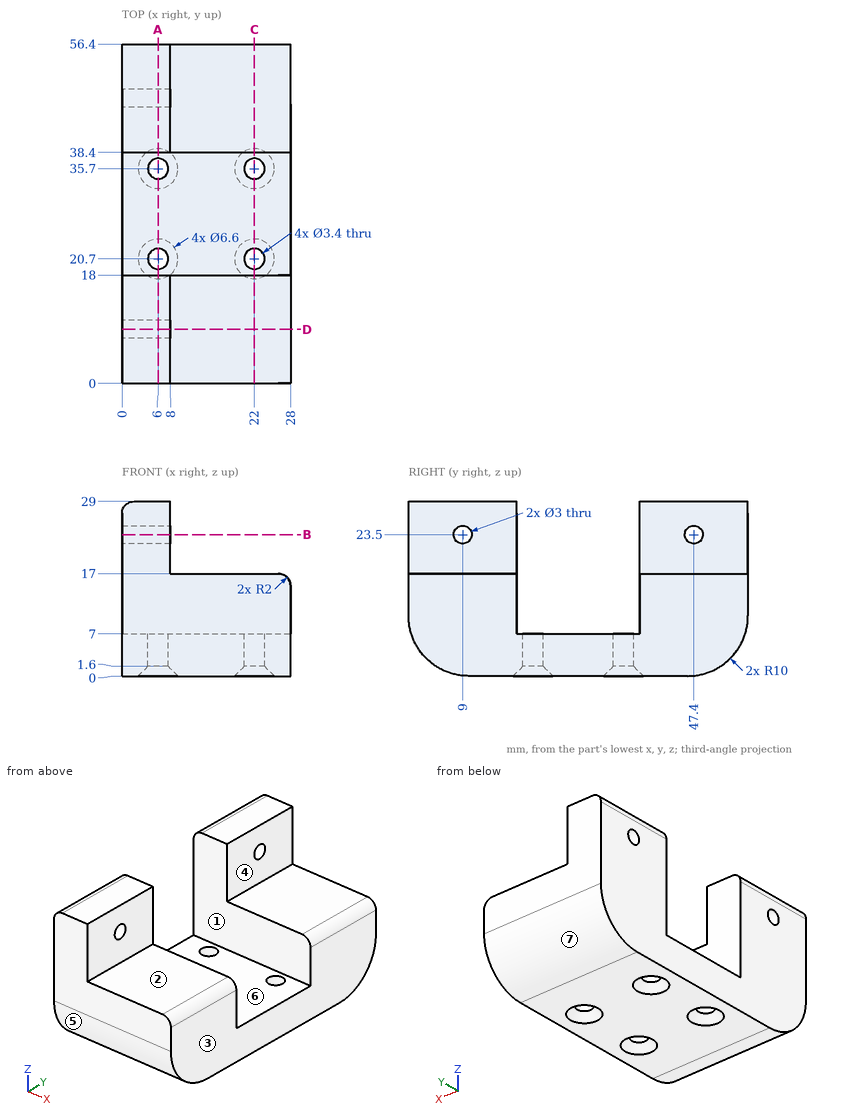
Drawing for the job (mm, zero at the part's lowest x, y, z). A direction names the side the tool comes from. Round coordinates to 2 decimals unless told otherwise and drop trailing zeros. Write each loop counter-clockwise with the first axis right and the second up, starting at its lowest first coordinate (ties: lowest second). Pieces come first, ordered by that corner, then holes. Notation, with made-up numbers: M 74.5,49 L 128.5,49 A7 ccw 128.5,54 Z; hole C 26,69.25 d2. An arc over 180 degrees is marked long. Put each result on its own line as item: value.
Item 1: Cut at D-D (y = 9). List the corners of the cut face in (x, z).
Responses:
outline: M 0,0.05 L 28,0.05 L 28,15 A2 ccw 26,17 L 8,17 L 8,22 L 0,22 Z; M 0,25 L 8,25 L 8,29 L 2,29 A2 ccw 0,27 Z
Item 2: Tool access for the marked faces 1, 2 and 3: list every direction of +Z, -Z, +X, -X, +Y, -Y with a clear straight run to the whole face (end or side of a thin tool).
Responses:
face 1: +Z, +X, -X
face 2: +Z, +X, +Y, -Y
face 3: +Z, -Z, +X, +Y, -Y
Item 3: Cut at A-A (x = 6). List the corners of the cut face in (y, z), and give its area (3 significant figures).
Responses:
outline: M 0,10 A10 ccw 10,0 L 17.4,0 L 19,1.6 L 19,7 L 18,7 L 18,29 L 0,29 Z; M 22.4,1.6 L 24,0 L 32.4,0 L 34,1.6 L 34,7 L 22.4,7 Z; M 37.4,1.6 L 39,0 L 46.4,0 A10 ccw 56.4,10 L 56.4,29 L 38.4,29 L 38.4,7 L 37.4,7 Z; hole C 9,23.5 d3; hole C 47.4,23.5 d3
area: 1,080 mm²
Item 4: Flat gauge pins, fed straight in: P1, Ø1.5, axis at x = 18.5, y = 8.5, coming from the -Z side; P2, Ø1.5, axis at x = 15.5, y = 13, coming from the +Z side; P3, Ø3, axis at x = 6, y = 35.7, coming from the -Z side; P4, Ø3.5, axis at y = 11.5, z = 21, coming from the +X side. Where does each tip first touch, or does it go through?
Responses:
P1: z = 0.03
P2: z = 17
P3: through
P4: x = 8
Item 5: Cut at B-B (z = 23.5). List the corners of the cut face in (x, y).
Responses:
outline: M 0,0 L 8,0 L 8,7.5 L 0,7.5 Z; M 0,10.5 L 8,10.5 L 8,18 L 0,18 Z; M 0,38.4 L 8,38.4 L 8,45.9 L 0,45.9 Z; M 0,48.9 L 8,48.9 L 8,56.4 L 0,56.4 Z
Item 6: Probe L1, parallel to X at y = 20.7, z = 2.8; L2, parallel to Y at x = 6.25, z = 23.5; L3, parallel to Y at x = 22, z = 3.75. List the from-to ranges inside material, lowest first. Write a range as from..to.
Responses:
L1: 0..4.3, 7.7..20.3, 23.7..28
L2: 0..7.5, 10.5..18, 38.4..45.9, 48.9..56.4
L3: 2.19..19, 22.4..34, 37.4..54.21
Item 7: Cut at C-C (x = 22). List the corners of the cut face in (y, z).
Responses:
outline: M 0,10 A10 ccw 10,0 L 17.4,0 L 19,1.6 L 19,7 L 18,7 L 18,17 L 0,17 Z; M 22.4,1.6 L 24,0 L 32.4,0 L 34,1.6 L 34,7 L 22.4,7 Z; M 37.4,1.6 L 39,0 L 46.4,0 A10 ccw 56.4,10 L 56.4,17 L 38.4,17 L 38.4,7 L 37.4,7 Z
Item 8: Mould opens along Y. For the marked faces 4, 5, 6 and 7 say: +Y half, -Y half, draft (parallel to the pull), parting line (faces both ways), or undercut.
Responses:
face 4: draft
face 5: -Y half
face 6: undercut
face 7: +Y half
